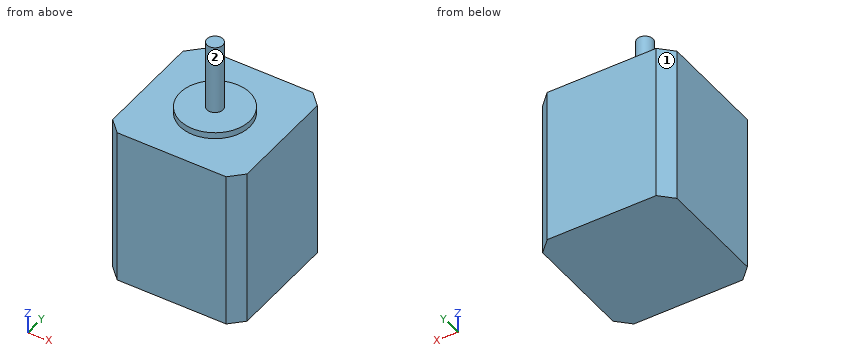
```python
from build123d import *

# Parameters (mm, degrees)
SKETCH_W        = 42.3
SKETCH_H        = 42.3
PAD_DEPTH       = 50
SKETCH001_R     = 11
PAD001_DEPTH    = 2
SKETCH002_R     = 2.5
PAD002_DEPTH    = 22
CHAMFER_SIZE    = 4
CHAMFER001_SIZE = 4
CHAMFER002_SIZE = 4
CHAMFER003_SIZE = 4


with BuildPart() as part:
    # Sketch → Pad (new body)
    with BuildSketch(Plane.XY):
        Rectangle(SKETCH_W, SKETCH_H)
    extrude(amount=PAD_DEPTH)

    # Sketch001 → Pad001 (new body)
    with BuildSketch(Plane.XY.offset(50)):
        Circle(SKETCH001_R)
    extrude(amount=PAD001_DEPTH)

    # Sketch002 → Pad002 (new body)
    with BuildSketch(Plane.XY.offset(52)):
        Circle(SKETCH002_R)
    extrude(amount=PAD002_DEPTH)

    # Chamfer
    chamfer_edges = [part.edges().sort_by_distance(p)[0] for p in [
        (-21.15, -21.15, 25),
    ]]
    chamfer(chamfer_edges, length=CHAMFER_SIZE)

    # Chamfer001
    chamfer001_edges = [part.edges().sort_by_distance(p)[0] for p in [
        (-21.15, 21.15, 25),
    ]]
    chamfer(chamfer001_edges, length=CHAMFER001_SIZE)

    # Chamfer002
    chamfer002_edges = [part.edges().sort_by_distance(p)[0] for p in [
        (21.15, 21.15, 25),
    ]]
    chamfer(chamfer002_edges, length=CHAMFER002_SIZE)

    # Chamfer003
    chamfer003_edges = [part.edges().sort_by_distance(p)[0] for p in [
        (21.15, -21.15, 25),
    ]]
    chamfer(chamfer003_edges, length=CHAMFER003_SIZE)


solid = part.part
```
Verification items for the finished model (mm, model axes). Face numbers are marked on the shaded views. A direction names the side the tool comes from. Round coordinates to 2 decimals unless told otherwise and drop trailing zeros. Write each loop counter-clockwise with the first axis right and the second up, starting at its lowest first coordinate (ties: lowest second). Pieces come first, ordered by that corner, then holes. Notation, with made-up numbers: (2.5, 22) - (25.5, 22) arc R7 cw to (25.5, 28) - close; hole circle Ø7 at (25, 28). An arc over 180 degrees is marked (long way). Answer as a JSON object with one key per item and string values. Group by question number.
Q1. Tool access check on the marked faces 1 and 2. Record the directions out of +Z, -Z, +X, -X, +Y, -Y that give a thin tool (end or side, any length) a straight path to the whole face; none if there is none.
Q2. Section check A-A, the plane x = 0. Enter the section's corners in (y, z), plus the area to 3 significant figures.
Q3. Section check B-B, the plane z = 20.5. Enter the section's corners in (x, y), plus the area to 3 significant figures.
Q4. Thickness scan on line 1 (Z direction, x = -2, y = 18.5); line 2 (Y direction, x = 0, z = 57.5); line 3 (Z direction, x = 2, y = 8.5). Record the ranges inside material, lowest first.
Q5. Section check D-D, the plane x = 9.5. Enter the section's corners in (y, z).
Found:
{
 "1": {"face 1": "+Z, -Z, -X, +Y", "face 2": "+Z"},
 "2": {"outline": "(-21.15, 0) - (21.15, 0) - (21.15, 50) - (11, 50) - (11, 52) - (2.5, 52) - (2.5, 74) - (-2.5, 74) - (-2.5, 52) - (-11, 52) - (-11, 50) - (-21.15, 50) - close", "area": "2,270 mm^2"},
 "3": {"outline": "(-21.15, -17.15) - (-17.15, -21.15) - (17.15, -21.15) - (21.15, -17.15) - (21.15, 17.15) - (17.15, 21.15) - (-17.15, 21.15) - (-21.15, 17.15) - close", "area": "1,760 mm^2"},
 "4": {"line 1": "z = 0 to 50", "line 2": "y = -2.5 to 2.5", "line 3": "z = 0 to 52"},
 "5": {"outline": "(-21.15, 0) - (21.15, 0) - (21.15, 50) - (5.55, 50) - (5.55, 52) - (-5.55, 52) - (-5.55, 50) - (-21.15, 50) - close"}
}
